from build123d import *

# Parameters (mm, degrees)
BOSS_EXTRUDE1_DEPTH = 70
BOSS_EXTRUDE3_REACH = 86.63
SKETCH3_W           = 1.8
SKETCH3_H           = 3.8
SKETCH4_W           = 5
SKETCH4_H           = 3
BOSS_EXTRUDE4_DEPTH = 2
CUT_EXTRUDE1_REACH  = 90.595
SKETCH5_R           = 1.5
SKETCH7_R           = 10
CUT_EXTRUDE2_DEPTH  = 85.630140132
BOSS_EXTRUDE5_DEPTH = 2
SKETCH10_R          = 4.358893906
CUT_EXTRUDE3_DEPTH  = 1.8
SKETCH9_R           = 1.5
BOSS_EXTRUDE6_DEPTH = 2
SKETCH11_W          = 10
SKETCH11_H          = 3
BOSS_EXTRUDE7_DEPTH = 3.5
SKETCH12_W          = 10
SKETCH12_H          = 15
BOSS_EXTRUDE8_DEPTH = 3
CUT_EXTRUDE4_REACH  = 82.96
SKETCH13_W          = 6.66
SKETCH13_H          = 4.15
CUT_EXTRUDE5_REACH  = 82.96
SKETCH15_R          = 1.8
CUT_EXTRUDE6_DEPTH  = 0.4
SKETCH17_W          = 2
SKETCH17_H          = 16.984057064
BOSS_EXTRUDE9_DEPTH = 5


with BuildPart() as part:
    # Sketch1 → Boss-Extrude1 (new body)
    with BuildSketch(Plane.XY):
        with BuildLine():
            Line((-30.398230088, 19.964424779), (-30.398230088, -13.495575221))
            ThreePointArc((-30.398230088, -13.495575221), (-28.708236216, -17.575581349), (-24.628230088, -19.265575221))
            Line((-24.628230088, -19.265575221), (9.601769912, -19.265575221))
            Line((9.601769912, -19.265575221), (9.601769912, -17.265575221))
            Line((9.601769912, -17.265575221), (-24.628230088, -17.265575221))
            ThreePointArc((-24.628230088, -17.265575221), (-27.294022654, -16.161367786), (-28.398230088, -13.495575221))
            Line((-28.398230088, -13.495575221), (-28.398230088, 19.964424779))
            ThreePointArc((-28.398230088, 19.964424779), (-27.294022654, 22.630217344), (-24.628230088, 23.734424779))
            Line((-24.628230088, 23.734424779), (-10.398230088, 23.734424779))
            Line((-10.398230088, 23.734424779), (-10.398230088, 25.734424779))
            Line((-10.398230088, 25.734424779), (-24.628230088, 25.734424779))
            ThreePointArc((-24.628230088, 25.734424779), (-28.708236216, 24.044430906), (-30.398230088, 19.964424779))
        make_face()
    extrude(amount=BOSS_EXTRUDE1_DEPTH)

    # Sketch3 → Boss-Extrude3 (add, up to next)
    with BuildSketch(Plane(origin=(9.601769912, 0, 0), x_dir=(0, 0, -1), z_dir=(1, 0, 0)), mode=Mode.PRIVATE) as boss_extrude3_sk1:
        with Locations((-69.1, -15.365575221)):
            Rectangle(SKETCH3_W, SKETCH3_H)
    boss_extrude3_tool1 = extrude(boss_extrude3_sk1.sketch, amount=-BOSS_EXTRUDE3_REACH, mode=Mode.PRIVATE) - part.part
    # Sketch3 → Boss-Extrude3 (add, up to next)
    with BuildSketch(Plane(origin=(9.601769912, 0, 0), x_dir=(0, 0, -1), z_dir=(1, 0, 0)), mode=Mode.PRIVATE) as boss_extrude3_sk2:
        with Locations((-0.9, -15.365575221)):
            Rectangle(SKETCH3_W, SKETCH3_H)
    boss_extrude3_tool2 = extrude(boss_extrude3_sk2.sketch, amount=-BOSS_EXTRUDE3_REACH, mode=Mode.PRIVATE) - part.part
    add(boss_extrude3_tool1.solids().sort_by_distance((9.60177, -15.365575, 69.1))[0])
    add(boss_extrude3_tool2.solids().sort_by_distance((9.60177, -15.365575, 0.9))[0])

    # Sketch4 → Boss-Extrude4 (add)
    with BuildSketch(Plane(origin=(0, -13.465575221, 0), x_dir=(1, 0, 0), z_dir=(0, 1, 0))):
        with Locations((7.101769912, -68.5)):
            Rectangle(SKETCH4_W, SKETCH4_H)
        with Locations((7.101769912, -1.5)):
            Rectangle(SKETCH4_W, SKETCH4_H)
    extrude(amount=BOSS_EXTRUDE4_DEPTH)

    # Sketch5 → Cut-Extrude1 (cut, up to next)
    with BuildSketch(Plane(origin=(0, -19.265575221, 0), x_dir=(-1, 0, 0), z_dir=(0, -1, 0)), mode=Mode.PRIVATE) as cut_extrude1_sk1:
        with Locations(Location((17.128230088, -60, 0), (0, 0, 180))):
            Circle(SKETCH5_R)
    cut_extrude1_tool1 = extrude(cut_extrude1_sk1.sketch, amount=-CUT_EXTRUDE1_REACH, mode=Mode.PRIVATE) & part.part
    # Sketch5 → Cut-Extrude1 (cut, up to next)
    with BuildSketch(Plane(origin=(0, -19.265575221, 0), x_dir=(-1, 0, 0), z_dir=(0, -1, 0)), mode=Mode.PRIVATE) as cut_extrude1_sk2:
        with Locations(Location((17.128230088, -10, 0), (0, 0, 90))):
            Circle(SKETCH5_R)
    cut_extrude1_tool2 = extrude(cut_extrude1_sk2.sketch, amount=-CUT_EXTRUDE1_REACH, mode=Mode.PRIVATE) & part.part
    # Sketch5 → Cut-Extrude1 (cut, up to next)
    with BuildSketch(Plane(origin=(0, -19.265575221, 0), x_dir=(-1, 0, 0), z_dir=(0, -1, 0)), mode=Mode.PRIVATE) as cut_extrude1_sk3:
        with Locations(Location((-2.871769912, -51.67, 0), (0, 0, 180))):
            Circle(SKETCH5_R)
    cut_extrude1_tool3 = extrude(cut_extrude1_sk3.sketch, amount=-CUT_EXTRUDE1_REACH, mode=Mode.PRIVATE) & part.part
    # Sketch5 → Cut-Extrude1 (cut, up to next)
    with BuildSketch(Plane(origin=(0, -19.265575221, 0), x_dir=(-1, 0, 0), z_dir=(0, -1, 0)), mode=Mode.PRIVATE) as cut_extrude1_sk4:
        with Locations(Location((-2.871769912, -18.33, 0), (0, 0, 90))):
            Circle(SKETCH5_R)
    cut_extrude1_tool4 = extrude(cut_extrude1_sk4.sketch, amount=-CUT_EXTRUDE1_REACH, mode=Mode.PRIVATE) & part.part
    add(cut_extrude1_tool1.solids().sort_by_distance((-17.12823, -19.265575, 60))[0], mode=Mode.SUBTRACT)
    add(cut_extrude1_tool2.solids().sort_by_distance((-17.12823, -19.265575, 10))[0], mode=Mode.SUBTRACT)
    add(cut_extrude1_tool3.solids().sort_by_distance((2.87177, -19.265575, 51.67))[0], mode=Mode.SUBTRACT)
    add(cut_extrude1_tool4.solids().sort_by_distance((2.87177, -19.265575, 18.33))[0], mode=Mode.SUBTRACT)

    # Sketch7 → Cut-Extrude2 (cut, through all)
    with BuildSketch(Plane.ZY.offset(30.398230088)):
        with Locations(Location((55, 3.234424779, 0), (0, 0, 270))):
            Circle(SKETCH7_R)
    extrude(amount=-CUT_EXTRUDE2_DEPTH, mode=Mode.SUBTRACT)

    # Sketch8 → Boss-Extrude5 (add)
    with BuildSketch(Plane.ZY.offset(30.398230088)):
        with BuildLine():
            Line((52, -4.181773708), (52, -6.304967235))
            ThreePointArc((52, -6.304967235), (55, -6.765575221), (58, -6.304967235))
            Line((58, -6.304967235), (58, -4.181773708))
            ThreePointArc((58, -4.181773708), (55, 11.234424779), (52, -4.181773708))
        make_face()
    extrude(amount=-BOSS_EXTRUDE5_DEPTH)

    # Sketch10 → Cut-Extrude3 (cut)
    with BuildSketch(Plane(origin=(-28.398230088, 0, 0), x_dir=(0, 0, -1), z_dir=(1, 0, 0))):
        with Locations(Location((-55, 3.234424779, 0), (0, 0, 90))):
            Circle(SKETCH10_R)
    extrude(amount=-CUT_EXTRUDE3_DEPTH, mode=Mode.SUBTRACT)

    # Sketch9 → Boss-Extrude6 (add)
    with BuildSketch(Plane(origin=(-28.398230088, 0, 0), x_dir=(0, 0, -1), z_dir=(1, 0, 0))):
        with Locations(Location((-55, 9.734424779, 0), (0, 0, 89.999266045))):
            Circle(SKETCH9_R)
    extrude(amount=BOSS_EXTRUDE6_DEPTH)

    # Sketch11 → Boss-Extrude7 (add)
    with BuildSketch(Plane(origin=(-28.398230088, 0, 0), x_dir=(0, 0, -1), z_dir=(1, 0, 0))):
        with Locations((-55, 14.734424779)):
            Rectangle(SKETCH11_W, SKETCH11_H)
    extrude(amount=BOSS_EXTRUDE7_DEPTH)

    # Sketch12 → Boss-Extrude8 (add)
    with BuildSketch(Plane(origin=(-24.898230088, 0, 0), x_dir=(0, 0, -1), z_dir=(1, 0, 0))):
        with Locations((-55, 8.734424779)):
            Rectangle(SKETCH12_W, SKETCH12_H)
    extrude(amount=BOSS_EXTRUDE8_DEPTH)

    # Sketch13 → Cut-Extrude4 (cut, up to next)
    with BuildSketch(Plane(origin=(-21.898230088, 0, 0), x_dir=(0, 0, -1), z_dir=(1, 0, 0)), mode=Mode.PRIVATE) as cut_extrude4_sk1:
        with Locations((-55, 9.734424779)):
            Rectangle(SKETCH13_W, SKETCH13_H)
    cut_extrude4_tool1 = extrude(cut_extrude4_sk1.sketch, amount=-CUT_EXTRUDE4_REACH, mode=Mode.PRIVATE) & part.part
    add(cut_extrude4_tool1.solids().sort_by_distance((-21.89823, 9.734425, 55))[0], mode=Mode.SUBTRACT)

    # Sketch15 → Cut-Extrude5 (cut, up to next)
    with BuildSketch(Plane(origin=(-21.898230088, 0, 0), x_dir=(0, 0, -1), z_dir=(1, 0, 0)), mode=Mode.PRIVATE) as cut_extrude5_sk1:
        with Locations((-55, 4.234424779)):
            Circle(SKETCH15_R)
    cut_extrude5_tool1 = extrude(cut_extrude5_sk1.sketch, amount=-CUT_EXTRUDE5_REACH, mode=Mode.PRIVATE) & part.part
    add(cut_extrude5_tool1.solids().sort_by_distance((-21.89823, 4.234425, 55))[0], mode=Mode.SUBTRACT)

    # Sketch16 → Cut-Extrude6 (cut)
    with BuildSketch(Plane.ZY.offset(30.398230088)):
        with BuildLine():
            Line((54, 9.234424779), (54, 4.234424779))
            ThreePointArc((54, 4.234424779), (55, 3.234424779), (56, 4.234424779))
            Line((56, 4.234424779), (56, 9.234424779))
            ThreePointArc((56, 9.234424779), (55, 10.234424779), (54, 9.234424779))
        make_face()
        with BuildLine():
            ThreePointArc((51.990895344, 7.766880364), (55, -2.205967162), (58.009104656, 7.766880364))
            ThreePointArc((58.009104656, 7.766880364), (57.869100871, 8.459988538), (58.562209044, 8.599992323))
            ThreePointArc((58.562209044, 8.599992323), (55, -3.205967162), (51.437790956, 8.599992323))
            ThreePointArc((51.437790956, 8.599992323), (52.130899129, 8.459988538), (51.990895344, 7.766880364))
        make_face()
    extrude(amount=-CUT_EXTRUDE6_DEPTH, mode=Mode.SUBTRACT)

    # Sketch17 → Boss-Extrude9 (add)
    with BuildSketch(Plane(origin=(0, -17.265575221, 0), x_dir=(1, 0, 0), z_dir=(0, 1, 0))):
        with Locations((-11.228230088, -35)):
            Rectangle(SKETCH17_W, SKETCH17_H)
    extrude(amount=BOSS_EXTRUDE9_DEPTH)


solid = part.part
The listing builds one solid part. Answer for the finished solid, in the listing's coordinates (mm). A direction names the side the tool comes from. Round coordinates to 2 decimals unless told otherwise and drop trailing zeros. Write each loop counter-clockwise with the first axis right and the second up, starting at its lowest first coordinate (ties: lowest second). Pieces come first, ordered by that corner, then holes. Notation, with made-up numbers: M 37,73.5 L 89,73.5 A25 ccw 89,102.5 Z; hole C 49.5,18.25 d9. An arc over 180 degrees is marked long. Write each question's results on one line, items separated by ' | '. Start each with the question number.
(1) The part is cut by section A-A, the plane x = -23.5. Write down the section's boundary in (y, z).
(2) The part is cut by section C-C, the plane z = 29. Write down the section's boundary in (x, y), and give its area (3 significant figures).
(3) Each of these flat-tipped pins is pushed along its axis until it touches: P1, Ø4, axis at y = -15, z = 36.5, coming from the -X side; P2, Ø3.5, axis at x = -24, y = 9, coming from the +Z side; P3, Ø2.5, axis at x = -24, y = 10.5, coming from the -Z side; P4, Ø1.5, axis at y = -5.5, z = 47.5, coming from the +X side. Where does it stop, or does it pass through?
(4) The part is cut by section B-B, the plane z = 10. Write down the section's boundary in (x, y).
(5) Find the intervals of material crossed by line 1 (Y direction, x = -23.65, z = 55); line 2 (Y direction, x = -22, z = 52); line 3 (Y direction, x = -16, z = 45.5), in increasing order.
(6) The part is cut by section D-D, the plane x = 5.5. Write down the section's boundary in (y, z), and give its area (3 significant figures).
(7) Determine the mould class of faces 1 (the flat face through (-18, 23.734, 35)), 2 (the flat face through (-7, -17.266, 35)), 3 (the cylindrical face through (-27.41, 8.54, 54.09)) for opening direction Z: +Z half, -Z half, draft (parallel to the pull), parting line (faces both ways), or undercut.
(8) For faces 4 (the cylindrical face through (-30.201, -2.202, 54.805)), 5 (the flat face through (-23, 11.809, 55)), 6 (the flat face through (-11, -15, 26.508)), determine the directions among +Z, -Z, +X, -X, +Y, -Y from which every point of the face is accessible in a straight line to the end or side of a thin tool.
Worked answers:
1) outline: M -19.27,0 L -13.47,0 L -13.47,1.8 L -17.27,1.8 L -17.27,68.2 L -13.47,68.2 L -13.47,70 L -19.27,70 Z; M 1.23,50 L 16.23,50 L 16.23,60 L 1.23,60 Z; M 23.73,0 L 25.73,0 L 25.73,70 L 23.73,70 Z; hole C 4.23,55 d3.6; hole M 7.66,51.67 L 11.81,51.67 L 11.81,58.33 L 7.66,58.33 Z
2) outline: M -30.4,-13.5 A5.77 ccw -24.63,-19.27 L 9.6,-19.27 L 9.6,-17.27 L -10.23,-17.27 L -10.23,-12.27 L -12.23,-12.27 L -12.23,-17.27 L -24.63,-17.27 A3.77 cw -28.4,-13.5 L -28.4,19.96 A3.77 cw -24.63,23.73 L -10.4,23.73 L -10.4,25.73 L -24.63,25.73 A5.77 ccw -30.4,19.96 Z | area: 204 mm²
3) P1: stops at x = -30.4 | P2: stops at z = 60 | P3: stops at z = 50 | P4: stops at x = -28.4
4) outline: M -30.4,-13.5 A5.77 ccw -24.63,-19.27 L -18.63,-19.27 L -18.63,-17.27 L -24.63,-17.27 A3.77 cw -28.4,-13.5 L -28.4,19.96 A3.77 cw -24.63,23.73 L -10.4,23.73 L -10.4,25.73 L -24.63,25.73 A5.77 ccw -30.4,19.96 Z; M -15.63,-19.27 L 9.6,-19.27 L 9.6,-17.27 L -15.63,-17.27 Z
5) line 1: y = -19.27 to -17.27, 1.23 to 2.43, 6.03 to 7.66, 11.81 to 16.23, 23.73 to 25.73 | line 2: y = -19.27 to -17.27, 1.23 to 7.66, 11.81 to 16.23, 23.73 to 25.73 | line 3: y = -19.27 to -17.27, 23.73 to 25.73
6) outline: M -19.27,0 L -11.47,0 L -11.47,3 L -13.47,3 L -13.47,1.8 L -17.27,1.8 L -17.27,68.2 L -13.47,68.2 L -13.47,67 L -11.47,67 L -11.47,70 L -19.27,70 Z | area: 166 mm²
7) face 1: draft | face 2: undercut | face 3: parting line
8) face 4: -X | face 5: +X, -X | face 6: +X
